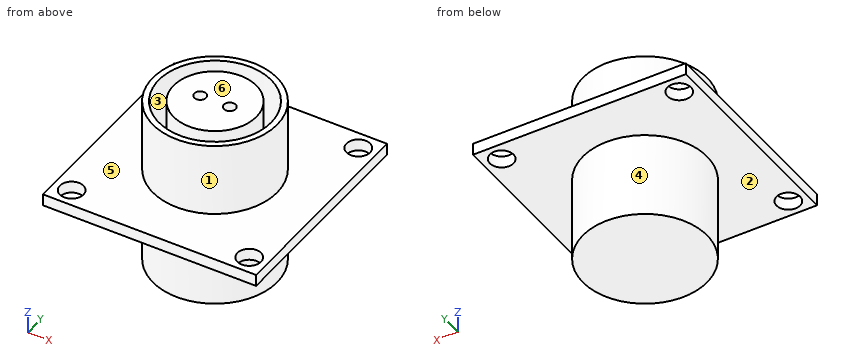
```python
from build123d import *

# Parameters (mm, degrees)
SKETCH_1_W           = 36
SKETCH_1_H           = 36
SKETCH_1_R           = 2
EXTRUDE_1_DEPTH      = 2
EXTRUDE_2_DEPTH      = 12.4
EXTRUDE_2_DEPTH_BACK = 16.4
SKETCH_2_R           = 10.5
SKETCH_3_R           = 9.5
SKETCH_3_R_2         = 7
SKETCH_3_R_3         = 1
CUT_EXTRUDE_1_DEPTH  = 10


with BuildPart() as part:
    # 草图1 → 凸台-拉伸1 (new body)
    with BuildSketch(Plane.XY):
        with Locations((15, -15)):
            Rectangle(SKETCH_1_W, SKETCH_1_H)
        Circle(SKETCH_1_R, mode=Mode.SUBTRACT)
        with Locations((0, -30)):
            Circle(SKETCH_1_R, mode=Mode.SUBTRACT)
        with Locations((30, -30)):
            Circle(SKETCH_1_R, mode=Mode.SUBTRACT)
        with Locations((30, 0)):
            Circle(SKETCH_1_R, mode=Mode.SUBTRACT)
    extrude(amount=EXTRUDE_1_DEPTH)

    # 草图2 → 凸台-拉伸2 (add, two sides: drawn at the far end of the back side and taken through both)
    with BuildSketch(Plane.XY.offset(2).offset(-EXTRUDE_2_DEPTH_BACK)):
        with Locations((15, -15)):
            Circle(SKETCH_2_R)
    extrude(amount=EXTRUDE_2_DEPTH + EXTRUDE_2_DEPTH_BACK)

    # 草图3 → 切除-拉伸1 (cut)
    # profile 1 of 3: a face of its own
    with BuildSketch(Plane.XY.offset(14.4)):
        with Locations((15, -15)):
            Circle(SKETCH_3_R)
        with Locations((15, -15)):
            Circle(SKETCH_3_R_2, mode=Mode.SUBTRACT)
    # profile 2 of 3: a face of its own
    with BuildSketch(Plane.XY.offset(14.4)):
        with Locations((17.5, -15)):
            Circle(SKETCH_3_R_3)
    # profile 3 of 3: a face of its own
    with BuildSketch(Plane.XY.offset(14.4)):
        with Locations((12.5, -15)):
            Circle(SKETCH_3_R_3)
    extrude(amount=-CUT_EXTRUDE_1_DEPTH, mode=Mode.SUBTRACT)


solid = part.part
```
Here's how the part is built. I have some questions about the finished solid (model axes, mm). Face numbers are marked on the shaded views. A direction names the side the tool comes from. Give positions to 0.01 mm unless a question says otherwise; leave off trailing zeros. Loops run counter-clockwise (first coordinate to the right, second up) from the corner with the lowest first, then second, coordinate; pieces in that order, holes last. Notation, with made-up numbers: M 85.25,-30.5 L 97.25,-30.5 A17 cw 97.25,-3.5 Z; hole C 53.25,64 d11. An arc over 180 degrees is marked long. Use one line per item in the form item = value. Start each with the question number.
Q1. If we section it at C-C (z = 9.25): Write out the boundary of the cut face in (x, y), then the cut area to 3 significant figures.
Q2. If we section it at A-A (x = 0): Write out the boundary of the cut face in (y, z), then the cut area to 3 significant figures.
Q3. Will these pins go through, and if not, where does the flat tip stop? pin 1 Ø5 at (x, z) = (26.5, -8.5) entering from -Y; pin 2 Ø12 at (x, z) = (20, 9) entering from +Y; pin 3 Ø3.5 at (x, y) = (0, 0) entering from -Z; pin 4 Ø12 at (y, z) = (-18, -6.5) entering from -X.
Q4. If we section it at D-D (x = 15): Write out the boundary of the cut face in (y, z), then the cut area to 3 significant figures.
Q5. Which directions (+Z, -Z, +X, -X, +Y, -Y) give clear straight access to the entire face, cutting with the end or side of a thin tool? Please do the marked faces 4, 5 and 6.
Q6. I need wall thicknesses on line 1 along Y through (x, z) = (30, 0.65); line 2 along Y through (x, z) = (15, 9.5); line 3 along X through (y, z) = (-29, 0.5). Which ranges of each line are inside material? Lowest first, please.
Q7. If we section it at B-B (y = -30): Write out the boundary of the cut face in (x, z), then the cut area to 3 significant figures.
Q8. Thinking about a two-plate mould opening in X: for the marked faces 1, 2 and 3, which applies, +X half, -X half, draft (parallel to the pull), parting line (faces both ways), or undercut?
Taken from the geometry:
q1.outline = C 15,-15 d21; C 15,-15 d14; hole C 15,-15 d19; hole C 12.5,-15 d2; hole C 17.5,-15 d2
q1.area = 210 mm^2
q2.outline = M -33,0 L -32,0 L -32,2 L -33,2 Z; M -28,0 L -2,0 L -2,2 L -28,2 Z; M 2,0 L 3,0 L 3,2 L 2,2 Z
q2.area = 56.0 mm^2
q3.pin_1 = -20.41
q3.pin_2 = -4.5
q3.pin_3 = through
q3.pin_4 = 4.5
q4.outline = M -33,0 L -25.5,0 L -25.5,-14.4 L -4.5,-14.4 L -4.5,0 L 3,0 L 3,2 L -4.5,2 L -4.5,14.4 L -5.5,14.4 L -5.5,4.4 L -8,4.4 L -8,14.4 L -22,14.4 L -22,4.4 L -24.5,4.4 L -24.5,14.4 L -25.5,14.4 L -25.5,2 L -33,2 Z
q4.area = 585 mm^2
q5.face_4 = -Z
q5.face_5 = +Z
q5.face_6 = +Z, +X, -X, +Y, -Y
q6.line_1 = -33 to -32, -28 to -2, 2 to 3
q6.line_2 = -25.5 to -24.5, -22 to -8, -5.5 to -4.5
q6.line_3 = -3 to -1.73, 1.73 to 28.27, 31.73 to 33
q7.outline = M -3,0 L -2,0 L -2,2 L -3,2 Z; M 2,0 L 28,0 L 28,2 L 2,2 Z; M 32,0 L 33,0 L 33,2 L 32,2 Z
q7.area = 56.0 mm^2
q8.face_1 = parting line
q8.face_2 = draft
q8.face_3 = undercut
